Can you work these out from the model? Positions are in its coordinate system, mm. A direction names the side the tool comes from. Give positions to 0.01 mm unless a question says otherwise; leave off trailing zeros. Loops run counter-clockwise (first coordinate to the right, second up) from the corner with the lowest first, then second, coordinate; pieces in that order, holes last. Notation, with made-up numbers: (16, 19) -> (75, 19) arc R16 ccw to (75, 32) -> close; hole circle Ø5 at (-2, 5). An arc over 180 degrees is marked (long way). One line per question, with ' | ' between items.
from build123d import *

# Parameters (mm, degrees)
SKETCH1_W           = 39.999999999
SKETCH1_H           = 30
BOSS_EXTRUDE1_DEPTH = 30
SKETCH2_W           = 14.6
SKETCH2_H           = 33.728920846
CUT_EXTRUDE1_DEPTH  = 25
SKETCH3_R           = 2.5
CUT_EXTRUDE2_DEPTH  = 77.38910698
SKETCH4_W           = 8.5
SKETCH4_H           = 4.5
SKETCH4_W_2         = 4.5
SKETCH4_H_2         = 8.5
CUT_EXTRUDE3_DEPTH  = 9
CUT_EXTRUDE4_START  = -40
SKETCH4_2_W         = 8.5
SKETCH4_2_H         = 4.5
SKETCH4_2_W_2       = 4.5
SKETCH4_2_H_2       = 8.5
CUT_EXTRUDE4_DEPTH  = 9
SKETCH5_R           = 2.5
CUT_EXTRUDE5_DEPTH  = 12
CHAMFER1_SIZE       = 4


with BuildPart() as part:
    # Sketch1 → Boss-Extrude1 (new body)
    with BuildSketch(Plane.XY):
        with Locations((-51.592932584, 42.752018711)):
            Rectangle(SKETCH1_W, SKETCH1_H)
    extrude(amount=BOSS_EXTRUDE1_DEPTH)

    # Sketch2 → Cut-Extrude1 (cut)
    with BuildSketch(Plane(origin=(0, 57.752018711, 0), x_dir=(1, 0, 0), z_dir=(0, 1, 0))):
        with Locations((-51.872932582, -8.135539577)):
            Rectangle(SKETCH2_W, SKETCH2_H)
    extrude(amount=-CUT_EXTRUDE1_DEPTH, mode=Mode.SUBTRACT)

    # Sketch3 → Cut-Extrude2 (cut, through all)
    with BuildSketch(Plane(origin=(-31.592932584, 0, 0), x_dir=(0, 0, -1), z_dir=(1, 0, 0))):
        with Locations((-12.822072937, 44.929945774)):
            Circle(SKETCH3_R)
    extrude(amount=-CUT_EXTRUDE2_DEPTH, mode=Mode.SUBTRACT)

    # Sketch4 → Cut-Extrude3 (cut)
    with BuildSketch(Plane(origin=(-31.592932584, 0, 0), x_dir=(0, 0, -1), z_dir=(1, 0, 0))):
        with Locations((-9.25, 35.002018711)):
            Rectangle(SKETCH4_W, SKETCH4_H)
        with Locations((-22.75, 48.502018711)):
            Rectangle(SKETCH4_W_2, SKETCH4_H_2)
    extrude(amount=-CUT_EXTRUDE3_DEPTH, mode=Mode.SUBTRACT)

    # Sketch4<2> → Cut-Extrude4 (cut)
    with BuildSketch(Plane(origin=(-31.592932584, 0, 0), x_dir=(0, 0, -1), z_dir=(1, 0, 0)).offset(CUT_EXTRUDE4_START)):
        with Locations((-9.25, 35.002018711)):
            Rectangle(SKETCH4_2_W, SKETCH4_2_H)
        with Locations((-22.75, 48.502018711)):
            Rectangle(SKETCH4_2_W_2, SKETCH4_2_H_2)
    extrude(amount=CUT_EXTRUDE4_DEPTH, mode=Mode.SUBTRACT)

    # Sketch5 → Cut-Extrude5 (cut)
    with BuildSketch(Plane.XY.offset(30)):
        with Locations((-66.592932583, 48.502018711)):
            Circle(SKETCH5_R)
        with Locations((-36.592932584, 48.502018711)):
            Circle(SKETCH5_R)
    cut_extrude5 = extrude(amount=-CUT_EXTRUDE5_DEPTH, mode=Mode.SUBTRACT)

    # Mirror1: Cut-Extrude5 across plane
    add(cut_extrude5.mirror(Plane(origin=(0, 28.876009355, 28.876009355), x_dir=(0, -0.7071067811865478, 0.7071067811865472), z_dir=(0, -0.7071067811865475, -0.7071067811865477))), mode=Mode.SUBTRACT)

    # Chamfer1
    chamfer1_edges = [part.edges().sort_by_distance(p)[0] for p in [
        (-51.592932584, 27.752018711, 30),
        (-65.382932583, 57.752018711, 0),
        (-51.592932584, 27.752018711, 0),
        (-38.082932583, 57.752018711, 0),
        (-51.592932584, 57.752018711, 30),
    ]]
    chamfer(chamfer1_edges, length=CHAMFER1_SIZE)


solid = part.part
Q1. If we section it at A-A (z = 9.25): State how many separate pieces and enclosed holes the cut face has, plus the area to 3 significant figures.
Entries:
separate pieces: 3 | enclosed holes: 0 | area: 679 mm²
Q2. For pin 1 Ø1.5 at (x, y) = (-56, 31.5) entering from -Z; pin 2 Ø2 at (y, z) = (35.5, 10.5) entering from +X; pin 3 Ø4 at (x, y) = (-36.59, 48.5) entering from +Z, each with a flat end and sliding along its axis, tell me the tip position at first contact or that it passes through.
Entries:
pin 1: z = 0 | pin 2: x = -40.59 | pin 3: z = 18
Q3. If we section it at D-D (y = 38.5): Write out the boundary of the cut face in (x, z).
Entries:
outline: (-71.59, 0) -> (-59.17, 0) -> (-59.17, 25) -> (-44.57, 25) -> (-44.57, 0) -> (-31.59, 0) -> (-31.59, 30) -> (-71.59, 30) -> close; hole circle Ø5 at (-66.59, 9.25); hole circle Ø5 at (-36.59, 9.25)
Q4. If we section it at B-B (y = 34.5): Write out the boundary of the cut face in (x, z).
Entries:
outline: (-71.59, 0) -> (-59.17, 0) -> (-59.17, 25) -> (-44.57, 25) -> (-44.57, 0) -> (-31.59, 0) -> (-31.59, 5) -> (-40.59, 5) -> (-40.59, 13.5) -> (-31.59, 13.5) -> (-31.59, 30) -> (-71.59, 30) -> (-71.59, 13.5) -> (-62.59, 13.5) -> (-62.59, 5) -> (-71.59, 5) -> close
Q5. If we mould it in two halves opening along X, with no side actions, what happens to faces 4 (the face through (-62.593, 35, 9)), 5 (the face through (-37.1, 30.2, 11.7)), 6 (the face through (-34, 49.4, 20.5))? For each: pulls with the +X half, pulls with the -X half, needs draft (parallel to the pull), parting line crosses it, or undercut.
Entries:
face 4: pulls with the -X half | face 5: undercut | face 6: needs draft
Q6. If I drill on probe 1 along Z at (x, y) = (-33, 45); probe 2 along X at (y, z) = (39.5, 8.5); probe 3 along X at (y, z) = (43, 14.5), over which ranges is the centre line in solid material (lowest first)? Write a range as from..to.
Entries:
probe 1: 0..10.32, 15.32..20.5, 25..30 | probe 2: -71.59..-68.98, -64.21..-59.17, -44.57..-38.98, -34.21..-31.59 | probe 3: -71.59..-59.17, -44.57..-31.59
Q7. On a 3-axis mill with a long thin cutter (end or side, diameter ignored), from which of +Z, -Z, +X, -X, +Y, -Y can I reach the whole of each face in a straight line? I mean faces 1 (the face through (-67, 44.252, 23)), 2 (the face through (-69.09, 48.61, 19.27)), 3 (the face through (-34, 32.752, 10)). Say none if no direction works.
Entries:
face 1: -X | face 2: +Z | face 3: +X
